```python
from build123d import *

# Parameters (mm, degrees)
SKETCH_1_W                = 45
SKETCH_1_H                = 48
EXTRUDE_1_DEPTH           = 12
SKETCH_2_R                = 6.5
CUT_EXTRUDE_1_DEPTH       = 12
HOLE_WIZARD_1_D           = 5.5
HOLE_WIZARD_1_CBORE_D     = 9.5
HOLE_WIZARD_1_CBORE_DEPTH = 30
SKETCH_14_R               = 3
CUT_EXTRUDE_2_DEPTH       = 8


with BuildPart() as part:
    # 草图1 → 凸台-拉伸1 (new body)
    with BuildSketch(Plane(origin=(0, 0, 0), x_dir=(1, 0, 0), z_dir=(0, 1, 0))):
        with Locations((22.5, 24)):
            Rectangle(SKETCH_1_W, SKETCH_1_H)
    extrude(amount=EXTRUDE_1_DEPTH)

    # 草图2 → 切除-拉伸1 (cut)
    with BuildSketch(Plane(origin=(0, 12, 0), x_dir=(1, 0, 0), z_dir=(0, 1, 0))):
        with Locations(Location((22.5, 25, 0), (0, 0, 270))):
            Circle(SKETCH_2_R)
    extrude(amount=-CUT_EXTRUDE_1_DEPTH, mode=Mode.SUBTRACT)

    # 打孔尺寸根据内六角圆柱头螺钉的类型1 (through all)
    with Locations(Plane(origin=(0, 0, -48), x_dir=(-1, 0, 0), z_dir=(0, 0, -1))):
        with Locations((-38.5, 6), (-6.5, 6)):
            CounterBoreHole(HOLE_WIZARD_1_D / 2, HOLE_WIZARD_1_CBORE_D / 2, HOLE_WIZARD_1_CBORE_DEPTH)

    # 草图14 → 切除-拉伸2 (cut)
    with BuildSketch(Plane.XZ):
        with Locations(Location((14.5, -43, 0), (0, 0, 270))):
            Circle(SKETCH_14_R)
        with Locations(Location((30.5, -43, 0), (0, 0, 270))):
            Circle(SKETCH_14_R)
    extrude(amount=-CUT_EXTRUDE_2_DEPTH, mode=Mode.SUBTRACT)


solid = part.part
```
Here's how the part is built. I have some questions about the finished solid (model axes, mm). A direction names the side the tool comes from. Coordinates: 2 decimals unless noted, no trailing zeros. Loops run counter-clockwise (first coordinate to the right, second up) from the corner with the lowest first, then second, coordinate; pieces in that order, holes last. Notation, with made-up numbers: M 7,24 L 58,24 A11 ccw 58,41 Z; hole C 1.5,79 d3. An arc over 180 degrees is marked long. One line per item, written item: value.
1. Will these pins go through, and if not, where does the flat tip stop? pin 1 Ø3 at (x, y) = (38.5, 6.5) entering from -Z; pin 2 Ø1.8 at (x, z) = (32, -43) entering from -Y; pin 3 Ø6.5 at (x, y) = (38.5, 6) entering from -Z.
Geometry says:
pin 1: passes through
pin 2: stops at y = 8
pin 3: stops at z = -18
2. Imagine slicing it at B-B (z = -29.5). List the corners of the cut face in (x, y) for me, and give its area (3 significant figures).
Geometry says:
outline: M 0,0 L 17.81,0 L 17.81,12 L 0,12 Z; M 27.19,0 L 45,0 L 45,12 L 27.19,12 Z; hole C 6.5,6 d9.5; hole C 38.5,6 d9.5
area: 286 mm2
3. On a 3-axis mill with a long thin cutter (end or side, diameter ignored), from which of +Z, -Z, +X, -X, +Y, -Y can I reach the whole of each face in a straight line? I mean faces 5 (the flat face through (36, 4, -18)), 6 (the flat face through (17, 0, -30)), 7 (the cylindrical face through (12.7, 3.9, -40.6)). Say none if no direction works.
Geometry says:
face 5: -Z
face 6: +Z, -Z, +X, -X, -Y
face 7: -Y
4. Imagine slicing it at A-A (y = 6). List the corners of the cut face in (x, z) for me, and give its area (3 significant figures).
Geometry says:
outline: M 0,-48 L 1.75,-48 L 1.75,-18 L 3.75,-18 L 3.75,0 L 0,0 Z; M 9.25,-18 L 11.25,-18 L 11.25,-48 L 33.75,-48 L 33.75,-18 L 35.75,-18 L 35.75,0 L 9.25,0 Z; M 41.25,-18 L 43.25,-18 L 43.25,-48 L 45,-48 L 45,0 L 41.25,0 Z; hole C 14.5,-43 d6; hole C 22.5,-25 d13; hole C 30.5,-43 d6
area: 1,200 mm2
5. Imagine slicing it at D-D (z = -35.5). List the corners of the cut face in (x, y) for me.
Geometry says:
outline: M 0,0 L 45,0 L 45,12 L 0,12 Z; hole C 6.5,6 d9.5; hole C 38.5,6 d9.5
6. Thinking about a two-plate mould opening in X: for faces 1 (the cylindrical face through (30.6, 3.9, -40)), 2 (the flat face through (22, 6, -48)), 3 (the flat face through (0, 6, -24)), 4 (the flat face through (45, 6, -24)), which applies, +X half, -X half, draft (parallel to the pull), parting line (faces both ways), or undercut?
Geometry says:
face 1: undercut
face 2: draft
face 3: -X half
face 4: +X half
7. Please list where these lines run through material, in increasing order: probe 1 along X at (y, z) = (2, -43); probe 2 along Y at (x, z) = (6.5, -9); probe 3 along X at (y, z) = (9.5, -38).
Geometry says:
probe 1: x = 0 to 3.94, 9.06 to 11.5, 17.5 to 27.5, 33.5 to 35.94, 41.06 to 45
probe 2: y = 0 to 3.25, 8.75 to 12
probe 3: x = 0 to 3.29, 9.71 to 35.29, 41.71 to 45
8. Imagine slicing it at C-C (x = 6.5). List the corners of the cut face in (y, z) for me.
Geometry says:
outline: M 0,-48 L 1.25,-48 L 1.25,-18 L 3.25,-18 L 3.25,0 L 0,0 Z; M 8.75,-18 L 10.75,-18 L 10.75,-48 L 12,-48 L 12,0 L 8.75,0 Z
